Geometry check sheet. Reference: the model listing, model coordinates, mm. A direction names the side the tool comes from. Give positions to 0.01 mm unless a question says otherwise; leave off trailing zeros. Loops run counter-clockwise (first coordinate to the right, second up) from the corner with the lowest first, then second, coordinate; pieces in that order, holes last. Notation, with made-up numbers: (-27, -1.5) -> (17, -1.5) arc R12 cw to (17, 21.5) -> close; hole circle Ø7 at (31, 77). An arc over 180 degrees is marked (long way). Write item = value, one per line.
Autodesk Inventor part; units mm, degrees
ref_plane "YZ Plane" through (0, 0, 0) normal (1, 0, 0) x (0, 1, 0)
ref_plane "XZ Plane" through (0, 0, 0) normal (0, 1, 0) x (-1, 0, 0)
ref_plane "XY Plane" through (0, 0, 0) normal (0, 0, 1) x (1, 0, 0)
sketch "Sketch1" plane through (0, 0, 0) normal (0, 0, 1) x (1, 0, 0)
  line L0 (-139.7, 31.75) -> (139.7, 31.75)
  line L1 (139.7, 31.75) -> (139.7, -31.75)
  line L2 (139.7, -31.75) -> (-139.7, -31.75)
  line L3 (-139.7, -31.75) -> (-139.7, 31.75)
  point P0 (0, 0)
  point P1 (0, 31.75)
  point P2 (139.7, 0)
  dimension "d0" = 279.4
  dimension "d1" = 63.5
extrude "Extrusion1" add sketch "Sketch1" along normal blind 43.18
sketch "Sketch2" plane through (0, 0, 43.18) normal (0, 0, 1) x (1, 0, 0)
  line L0 (-139.7, -31.75) -> (139.7, -31.75)
  line L1 (-138.1125, 30.1625) -> (138.1125, 30.1625)
  line L2 (138.1125, 30.1625) -> (138.1125, -31.75)
  line L3 (138.1125, -31.75) -> (-138.1125, -31.75)
  line L4 (-138.1125, -31.75) -> (-138.1125, 30.1625)
  line L5 (139.7, -31.75) -> (139.7, 31.75)
  line L6 (139.7, 31.75) -> (-139.7, 31.75)
  line L7 (-139.7, 31.75) -> (-139.7, -31.75)
  point P0 (0, 0)
  point P1 (-138.1125, -31.75)
  dimension "d4" = 1.5875
  dimension "d5" = 1.5875
  dimension "d6" = 1.5875
extrude "Extrusion2" cut sketch "Sketch2" against normal up to surface (43.18 mm away) contours L4 L1 L2 L0
sketch "Sketch3" plane through (-138.1125, -31.75, 43.18) normal (1, 0, 0) x (0, 0, -1)
  circle A0 centre (21.59, 41.5925) radius 5.05
  line L0 (0, 61.9125) -> (43.18, 61.9125)
  circle A1 centre (21.59, 21.2725) radius 1.5875
  line L1 (43.18, 63.5) -> (0, 63.5)
  point P0 (43.18, 31.75)
  point P1 (21.59, 63.5)
  dimension "d9" = 10.1
  dimension "d10" = 20.32
  dimension "d13" = 3.175
  dimension "d15" = 20.32
extrude "Extrusion3" cut sketch "Sketch3" along normal through all both and the other way through all
sketch "Sketch4" plane through (139.7, -31.75, 0) normal (1, 0, 0) x (0, 0, -1)
  circle A0 centre (-10.16, 26.3525) radius 2.3813
  line L0 (0, 63.5) -> (-43.18, 63.5) construction
  line L1 (-21.59, 63.5) -> (-21.59, -3.1611) construction
  line L2 (0, 0) -> (0, 63.5)
  circle A1 centre (-21.59, 41.5925) radius 5.05
  circle A2 centre (-33.02, 26.3525) radius 2.3813
  point P0 (0, 31.75)
  dimension "d16" = 10.16
  dimension "d17" = 15.24
  dimension "d18" = 4.7625
extrude "Extrusion4" cut sketch "Sketch4" against normal up to surface (1.5875 mm away) contours A0 | A2
sketch "Sketch5" plane through (-139.7, -31.75, 0) normal (-1, 0, 0) x (0, 0, 1)
  circle A0 centre (21.59, 41.5925) radius 5.05 construction
  line L0 (21.59, 41.5925) -> (21.59, 66.4825) construction
  line L1 (21.59, 41.5925) -> (51.2225, 41.5925) construction
  circle A1 centre (37.09, 57.0925) radius 1.5875
  circle A2 centre (6.09, 57.0925) radius 1.5875
  circle A3 centre (37.09, 26.0925) radius 1.5875
  circle A4 centre (6.09, 26.0925) radius 1.5875
  point P0 (0, 31.75)
  dimension "d21" = 3.175
  dimension "d22" = 15.5
  dimension "d23" = 15.5
extrude "Extrusion5" cut sketch "Sketch5" against normal up to surface (1.5875 mm away)
sketch "Sketch6" plane through (0, 0, 43.18) normal (0, 0, 1) x (1, 0, 0)
  line L0 (-138.1125, 30.1625) -> (138.1125, 30.1625)
  line L1 (-138.1125, 30.1625) -> (155.4569, 30.1625)
  line L2 (155.4569, 30.1625) -> (155.4569, 53.3555)
  line L3 (155.4569, 53.3555) -> (-138.1125, 53.3555)
  line L4 (-138.1125, 53.3555) -> (-138.1125, 30.1625)
  line L5 (155.4569, 53.3555) -> (81.9347, 53.3555)
  line L6 (81.9347, 53.3555) -> (81.9347, -39.2964)
  line L7 (81.9347, -39.2964) -> (155.4569, -39.2964)
  line L8 (155.4569, -39.2964) -> (155.4569, 53.3555)
  line L9 (-138.1125, 30.1625) -> (-141.389, 30.1625)
  line L10 (-141.389, 30.1625) -> (-141.389, 34.0033)
  line L11 (-141.389, 34.0033) -> (-138.1125, 34.0033)
  line L12 (-138.1125, 34.0033) -> (-138.1125, 30.1625)
  point P0 (0, 0)
  point P1 (81.9347, 30.1625)
extrude "Extrusion6" cut sketch "Sketch6" against normal through all
sketch "Sketch7" plane through (-139.7, -31.75, 0) normal (-1, 0, 0) x (0, 0, 1)
  line L0 (43.18, 61.9125) -> (0, 61.9125)
  line L1 (0, 61.9125) -> (0, 0)
  line L2 (0, 0) -> (43.18, 0)
  line L3 (43.18, 61.9125) -> (43.18, 0)
  circle A0 centre (37.09, 26.0925) radius 1.5875
  circle A1 centre (6.09, 57.0925) radius 1.5875
  circle A2 centre (6.09, 26.0925) radius 1.5875
  circle A3 centre (37.09, 57.0925) radius 1.5875
  circle A4 centre (21.59, 41.5925) radius 5.05
  circle A5 centre (21.59, 21.2725) radius 1.5875
  point P0 (0, 31.75)
extrude "Extrusion7" add sketch "Sketch7" against normal blind 6.35
sketch "Sketch8" plane through (-139.7, 30.1625, 43.18) normal (0, 1, 0) x (1, 0, 0)
  line L0 (0, 0) -> (6.35, 0)
  line L1 (3.175, 0) -> (3.175, 11.43)
  line L2 (0, 43.18) -> (6.35, 43.18)
  line L3 (3.175, 43.18) -> (3.175, 31.75)
  point P0 (139.7, 43.18)
  dimension "d30" = 11.43
  dimension "d31" = 11.43
hole "Hole1" at (-136.525, 30.1625, 31.75) at (-136.525, 30.1625, 11.43) direction (0, -1, 0) diameter 2.6416 depth 10.9728 tip angle 118
properties part number "Bracket(left)"
Item 1: Section check C-C, the plane y = 6.5. Record the cut outline in (x, z), plus the area to 3 significant figures.
Answer:
outline = (-139.7, 0) -> (-133.35, 0) -> (-133.35, 17.8) -> (-139.7, 17.8) -> close; (-139.7, 25.38) -> (-133.35, 25.38) -> (-133.35, 43.18) -> (-139.7, 43.18) -> close
area = 226 mm^2
Item 2: Gauge pin test, flat ends, axial feed: pin 1 (4 mm diameter, centred on y = -10.48, z = 21.59, fed in from -X); pin 2 (2.5 mm diameter, centred on x = -136.525, z = 11.43, fed in from +Y). Record the tip position at first contact, or that the pin passes through.
Answer:
pin_1 = -139.7
pin_2 = 19.15
Item 3: Draft check along Z on faces 1 (the flat face through (-137, 0, 0)), 2 (the flat face through (-139.7, -1, 21)), 3 (the flat face through (-137, 0, 43.18)), 4 (the cylindrical face through (-136.569, -5.588, 35.504)). Enter one of: +Z half, -Z half, draft (parallel to the pull), parting line (faces both ways), or undercut.
Answer:
face_1 = -Z half
face_2 = draft
face_3 = +Z half
face_4 = undercut
Item 4: Section check B-B, the plane y = 26. Record the cut outline in (x, z) (3 decimals), plus the area to 3 significant figures.
Answer:
outline = (-139.7, 0) -> (-133.35, 0) -> (-133.35, 4.645) -> (-139.7, 4.645) -> close; (-139.7, 7.535) -> (-133.35, 7.535) -> (-133.35, 35.645) -> (-139.7, 35.645) -> close; (-139.7, 38.535) -> (-133.35, 38.535) -> (-133.35, 43.18) -> (-139.7, 43.18) -> close; hole circle Ø2.642 at (-136.525, 11.43); hole circle Ø2.642 at (-136.525, 31.75)
area = 227 mm^2
Item 5: Section check A-A, the plane z = 37.09. Give the number of separate pieces and of enclosed holes in the cut face, plus the area to 3 significant figures.
Answer:
separate_pieces = 3
enclosed_holes = 0
area = 353 mm^2
Item 6: Section check D-D, the plane z = 18. Record the cut outline in (x, y).
Answer:
outline = (-139.7, -31.75) -> (-133.35, -31.75) -> (-133.35, 6.29) -> (-139.7, 6.29) -> close; (-139.7, 13.39) -> (-133.35, 13.39) -> (-133.35, 30.16) -> (-139.7, 30.16) -> close
Item 7: Thickness scan on L1, parallel to Y at x = -134.5, z = 21; L2, parallel to Z at x = -134.75, y = 26; L3, parallel to Z at x = -138, y = 11. Record the ranges inside material, lowest first. Write a range as [from, to].
Answer:
L1 = [-31.75, -11.95], [-9, 4.83], [14.86, 30.16]
L2 = [0, 4.65], [7.53, 35.65], [38.53, 43.18]
L3 = [0, 16.67], [26.51, 43.18]
Item 8: Tool access check on faces 5 (the cylindrical face through (-137.835, 24.599, 11.258)), 6 (the flat face through (-136, -31.75, 21)). Record the directions out of +Z, -Z, +X, -X, +Y, -Y that give a thin tool (end or side, any length) a straight path to the whole face; none if there is none.
Answer:
face_5 = +Y
face_6 = +Z, -Z, +X, -X, -Y
